Geometry check sheet. Reference: drawing and pictorial views, mm from the part's lowest x, y, z. Give positions to 0.01 mm unless a question says otherwise; leave off trailing zeros. Order: outer loops, then holes, each group sorted by start corner. A loop starts at its lowest first (then second) coordinate and runs counter-clockwise, first axis right, second up.
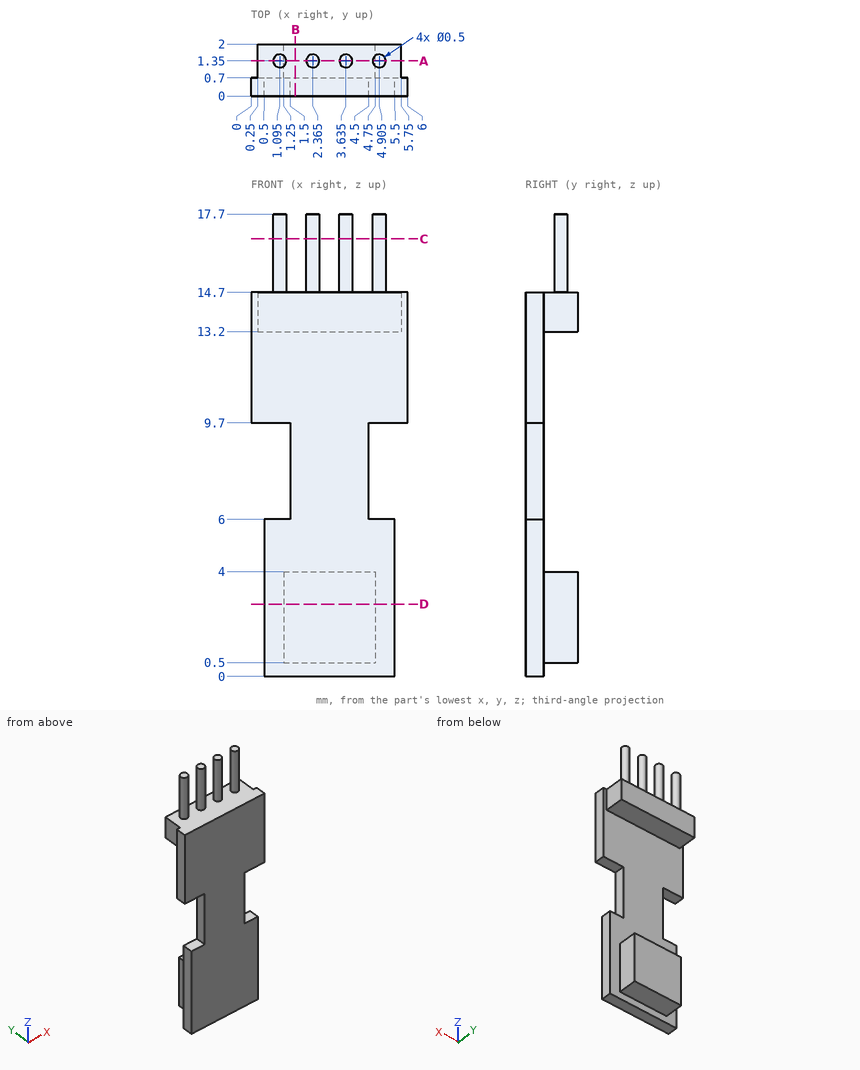
(1) Cross-section at D-D on z = 2.75. Enter the section's corners in (x, y), then the cut area to 3 significant figures.
Response values:
outline: (0.5, 0) - (5.5, 0) - (5.5, 0.7) - (4.75, 0.7) - (4.75, 2) - (1.25, 2) - (1.25, 0.7) - (0.5, 0.7) - close
area: 8.05 mm2
(2) Cross-section at B-B on x = 1.7. Enter the section's corners in (y, z), then the cut area to 3 significant figures.
Response values:
outline: (0, 0) - (0.7, 0) - (0.7, 0.5) - (2, 0.5) - (2, 4) - (0.7, 4) - (0.7, 13.2) - (2, 13.2) - (2, 14.7) - (0, 14.7) - close
area: 16.8 mm2
(3) Material ranges on L1, parallel to Z at x = 1.3, y = 1.3; L2, parallel to Z at x = 2.9, y = 1.45; L3, parallel to Y at x = 1.8, z = 6.5, recorded low to high.
Response values:
L1: z = 0.5 to 4, 13.2 to 17.7
L2: z = 0.5 to 4, 13.2 to 14.7
L3: y = 0 to 0.7
(4) Cross-section at C-C on z = 16.75. Enter the section's corners in (x, y) (3 decimals).
Response values:
outline: circle Ø0.5 at (1.095, 1.35); circle Ø0.5 at (2.365, 1.35); circle Ø0.5 at (3.635, 1.35); circle Ø0.5 at (4.905, 1.35)
(5) Gauge pin test, flat ends, axial feed: pin 1 Ø0.6 at (y, z) = (0, 3) entering from -X; pin 2 Ø1.8 at (x, z) = (2.5, 6) entering from +Y; pin 3 Ø1 at (y, z) = (1, 2) entering from +X. Record the tip position at first contact, or that the pin passes through.
Response values:
pin 1: stops at x = 0.5
pin 2: stops at y = 0.7
pin 3: stops at x = 5.5
(6) Cross-section at A-A on y = 1.35. Enter the section's corners in (x, z) (3 decimals).
Response values:
outline: (0.25, 13.2) - (5.75, 13.2) - (5.75, 14.7) - (5.155, 14.7) - (5.155, 17.7) - (4.655, 17.7) - (4.655, 14.7) - (3.885, 14.7) - (3.885, 17.7) - (3.385, 17.7) - (3.385, 14.7) - (2.615, 14.7) - (2.615, 17.7) - (2.115, 17.7) - (2.115, 14.7) - (1.345, 14.7) - (1.345, 17.7) - (0.845, 17.7) - (0.845, 14.7) - (0.25, 14.7) - close; (1.25, 0.5) - (4.75, 0.5) - (4.75, 4) - (1.25, 4) - close
